```python
from build123d import *

# Parameters (mm, degrees)
F0_W          = 400
F0_H          = 55.75
F2_W          = 20
F2_H          = 19.3462212823
F3_DEPTH      = 30
F4_R          = 15
F5_DEPTH      = 5
F7_DEPTH      = 13
F9_DEPTH      = 50
F11_DEPTH     = 12
F12_R         = 6
F13_DEPTH     = 40
F14_T1_DEPTH  = 63
F14_T3_DEPTH  = 10
F14_S7_W      = 5.1
F14_S7_H      = 5.1
F14_T8_DEPTH  = 5.1
F14_S13_W     = 5.1
F14_S13_H     = 5.1
F14_T14_DEPTH = 5.1
F14_T20_DEPTH = 51
F14_T25_DEPTH = 51


# Not quite as in the source:
# - a fillet or chamfer that OpenCascade refuses, or shapes differently, is made with other operations: its cross-section is extruded or revolved along the edge and cut away or added
# - a pattern or mirror of a feature is missing from the dataset's text; its kind, count and spacing are read off the source's solid


with BuildPart() as f1:
    # F0 (on Front) → F1 (revolve)
    with BuildSketch(Plane.XZ):
        with Locations((0, 27.875)):
            Rectangle(F0_W, F0_H)
        with BuildLine():
            ThreePointArc((200, 55.75), (0, 56.5), (-200, 55.75))
            Line((-200, 55.75), (200, 55.75))
        make_face()
    revolve(axis=Axis((0, 0, 0), (1, 0, 0)))

    # F2 (on face) → F3 (join)
    with BuildSketch(Plane(origin=(-200, 0, 0), x_dir=(0, -1, 0), z_dir=(-1, 0, 0))):
        Rectangle(F2_W, F2_H)
        with BuildLine():
            ThreePointArc((-10, -9.6731106412), (0, -12.5), (10, -9.6731106412))
            Line((10, -9.6731106412), (-10, -9.6731106412))
        make_face()
        with BuildLine():
            Line((-10, 9.6731106412), (10, 9.6731106412))
            ThreePointArc((10, 9.6731106412), (0, 12.5), (-10, 9.6731106412))
        make_face()
    f3 = extrude(amount=F3_DEPTH)

    # F3_copies: F3 across plane
    add(f3.mirror(Plane(origin=(0, 0, 0), x_dir=(0, 0, 1), z_dir=(1, 0, 0))))

    # F4 (on face) → F5 (join)
    with BuildSketch(Plane(origin=(-200, 0, 0), x_dir=(0, -1, 0), z_dir=(-1, 0, 0))):
        Circle(F4_R)
        with BuildLine():
            Line((10, 9.6731106412), (10, -9.6731106412))
            ThreePointArc((10, -9.6731106412), (0, -12.5), (-10, -9.6731106412))
            Line((-10, -9.6731106412), (-10, 9.6731106412))
            ThreePointArc((-10, 9.6731106412), (0, 12.5), (10, 9.6731106412))
        make_face(mode=Mode.SUBTRACT)
    f5 = extrude(amount=F5_DEPTH)

    # F5_copies: F5 across plane
    add(f5.mirror(Plane(origin=(0, 0, 0), x_dir=(0, 0, 1), z_dir=(1, 0, 0))))

    # F6 (on face) → F7 (join)
    with BuildSketch(Plane(origin=(-230, 0, 0), x_dir=(0, -1, 0), z_dir=(-1, 0, 0))):
        Polygon((10, 0.6794919243), (5.1961524227, 9), (-5.1961524227, 9), (-10, 0.6794919243), (-10, -0.6794919243), (-5.1961524227, -9), (5.1961524227, -9), (10, -0.6794919243), align=None)
    extrude(amount=F7_DEPTH)

    # F8 (on face) → F9 (join)
    with BuildSketch(Plane.XY.offset(9)):
        Polygon((-243, 10), (-269, 10), (-269, -10), (-243, -10), (-243, -5.1961524227), (-243, 5.1961524227), align=None)
    extrude(amount=-F9_DEPTH)

    # F10 (on face) → F11 (cut)
    with BuildSketch(Plane(origin=(0, 0, -41), x_dir=(1, 0, 0), z_dir=(0, 0, -1))):
        Polygon((-269, -10), (-259.1794919243, -10), (-267.5, -5.1961524227), (-267.5, 5.1961524227), (-259.1794919243, 10), (-269, 10), align=None)
        Polygon((-257.8205080757, -10), (-243, -10), (-243, 10), (-257.8205080757, 10), (-249.5, 5.1961524227), (-249.5, -5.1961524227), align=None)
    extrude(amount=-F11_DEPTH, mode=Mode.SUBTRACT)

    # F12 (on face) → F13 (join)
    with BuildSketch(Plane(origin=(0, 0, -41), x_dir=(1, 0, 0), z_dir=(0, 0, -1))):
        with Locations((-258.5, 0)):
            Circle(F12_R)
    extrude(amount=F13_DEPTH)

    # F14: fillet of radius 5 on 5 edges, made by hand

    # F14_s2 → F14_t1 (cut)
    with BuildSketch(Plane.XY.offset(-59)):
        with BuildLine():
            ThreePointArc((-269, -5), (-267.5355339059, -8.5355339059), (-264, -10))
            Line((-264, -10), (-264, -10.1))
            Line((-264, -10.1), (-269.1, -10.1))
            Line((-269.1, -10.1), (-269.1, -5))
            Line((-269.1, -5), (-269, -5))
        make_face()
        with BuildLine():
            ThreePointArc((-264, 10), (-267.5355339059, 8.5355339059), (-269, 5))
            Line((-269, 5), (-269.1, 5))
            Line((-269.1, 5), (-269.1, 10.1))
            Line((-269.1, 10.1), (-264, 10.1))
            Line((-264, 10.1), (-264, 10))
        make_face()
    extrude(amount=F14_T1_DEPTH, mode=Mode.SUBTRACT)

    # F14_s4 → F14_t3 (cut)
    with BuildSketch(Plane.XZ.offset(-5)):
        with BuildLine():
            ThreePointArc((-264, 9), (-267.5355339059, 7.5355339059), (-269, 4))
            Line((-269, 4), (-269.1, 4))
            Line((-269.1, 4), (-269.1, 9.1))
            Line((-269.1, 9.1), (-264, 9.1))
            Line((-264, 9.1), (-264, 9))
        make_face()
    extrude(amount=F14_T3_DEPTH, mode=Mode.SUBTRACT)


with BuildPart() as f14_tool6:
    # F14_s7 → F14_t8 (new body)
    with BuildSketch(Plane.XZ.offset(5)):
        with Locations((-266.55, 6.55)):
            Rectangle(F14_S7_W, F14_S7_H)
    extrude(amount=F14_T8_DEPTH)

    # F14_s9 → F14_t10 (revolve, cut)
    with BuildSketch(Plane(origin=(-264, -5, 4), x_dir=(0.7071067812, 0, -0.7071067812), z_dir=(-0.7071067812, 0, -0.7071067812))):
        with BuildLine():
            ThreePointArc((0, -5), (5, 0), (0, 5))
            Line((0, 5), (0, -5))
        make_face()
    revolve(axis=Axis((-264, -5, 4), (0, -1, 0)), mode=Mode.SUBTRACT)


with BuildPart() as f1_1:
    add(f1.part)

    # F14_t5: cut F14_tool6
    add(f14_tool6.part, mode=Mode.SUBTRACT)


with BuildPart() as f14_tool12:
    # F14_s13 → F14_t14 (new body)
    with BuildSketch(Plane.XZ.offset(-5)):
        with Locations((-266.55, 6.55)):
            Rectangle(F14_S13_W, F14_S13_H)
    extrude(amount=-F14_T14_DEPTH)

    # F14_s15 → F14_t16 (revolve, cut)
    with BuildSketch(Plane(origin=(-264, 5, 4), x_dir=(0.7071067812, 0, -0.7071067812), z_dir=(0.7071067812, 0, 0.7071067812))):
        with BuildLine():
            ThreePointArc((0, -5), (5, 0), (0, 5))
            Line((0, 5), (0, -5))
        make_face()
    revolve(axis=Axis((-264, 5, 4), (0, 1, 0)), mode=Mode.SUBTRACT)


with BuildPart() as f1_2:
    add(f1_1.part)

    # F14_t11: cut F14_tool12
    add(f14_tool12.part, mode=Mode.SUBTRACT)


with BuildPart() as f14_tool18:
    # F14_s19 → F14_t20 (new body)
    with BuildSketch(Plane.YZ.offset(-264)):
        with BuildLine():
            ThreePointArc((-5, 9), (-8.5355339059, 7.5355339059), (-10, 4))
            Line((-10, 4), (-10.1, 4))
            Line((-10.1, 4), (-10.1, 9.1))
            Line((-10.1, 9.1), (-5, 9.1))
            Line((-5, 9.1), (-5, 9))
        make_face()
    extrude(amount=F14_T20_DEPTH)

    split(bisect_by=Plane.YZ.offset(-230), keep=Keep.BOTTOM)


with BuildPart() as f1_3:
    add(f1_2.part)

    # F14_t17: cut F14_tool18
    add(f14_tool18.part, mode=Mode.SUBTRACT)


with BuildPart() as f14_tool23:
    # F14_s24 → F14_t25 (new body)
    with BuildSketch(Plane.YZ.offset(-213)):
        with BuildLine():
            ThreePointArc((10, 4), (8.5355339059, 7.5355339059), (5, 9))
            Line((5, 9), (5, 9.1))
            Line((5, 9.1), (10.1, 9.1))
            Line((10.1, 9.1), (10.1, 4))
            Line((10.1, 4), (10, 4))
        make_face()
    extrude(amount=-F14_T25_DEPTH)

    split(bisect_by=Plane.YZ.offset(-230), keep=Keep.BOTTOM)


with BuildPart() as f1_4:
    add(f1_3.part)

    # F14_t22: cut F14_tool23
    add(f14_tool23.part, mode=Mode.SUBTRACT)


solid = f1_4.part
```
Geometry check sheet. Reference: the model listing, model coordinates, mm. A direction names the side the tool comes from. Round coordinates to 2 decimals unless told otherwise and drop trailing zeros. Loops run counter-clockwise (first coordinate to the right, second up) from the corner with the lowest first, then second, coordinate; pieces in that order, holes last. Notation, with made-up numbers: (67, 15) -> (96, 15) arc R20 ccw to (96, 30) -> close; hole circle Ø3 at (31, 47.25). An arc over 180 degrees is marked (long way). Use a Markdown table: item, result.
(1) Mould release check, pull along X, two halves, no side actions. Record for faces 6 (the flat face through (230, 0, 0)), 7 (the flat face through (-247, 0, -29)), 8 (the flat face through (-269, 0, -12)), 9 (the flat face through (-259, 0, -81)): released by +X, released by -X, zero draft, split by the parting line, or undercut.
Calculated:
| item | result |
|---|---|
| face 6 | released by +X |
| face 7 | undercut |
| face 8 | released by -X |
| face 9 | zero draft |
(2) Sectioned sample at A-A (z = -65). Enter the section's corners in (x, y), then the cut area to 3 significant figures.
Calculated:
| item | result |
|---|---|
| outline | circle Ø12 at (-258.5, 0) |
| area | 113 mm² |
(3) Set-up check for faces 1 (the flat face through (-263.398, -7.564, -35.084)), 2 (the cylindrical face through (-252.777, -1.802, -60.72)), 3 (the flat face through (-236.409, -7.633, 4.78)), 4 (the flat face through (217, 10, 0)), 5 (the flat face through (-236.409, -7.564, -4.898)): record each of +Z, -Z, +X, -X, +Y, -Y from which the full face is reachable in a straight line by a thin tool's end or side.
Calculated:
| item | result |
|---|---|
| face 1 | -Z, -X, -Y |
| face 2 | -Z |
| face 3 | +Z, -Y |
| face 4 | +Z, -Z, +X, +Y |
| face 5 | -Z, -Y |
(4) Scan lines: probe 1 along X at (y, z) = (-3.5, -12); probe 2 along X at (y, z) = (42.5, -7); probe 3 along Y at (x, z) = (196, 0). Record each from-to range of solid material in increasing order.
Calculated:
| item | result |
|---|---|
| probe 1 | -269 to -243, -230 to 230 |
| probe 2 | -200 to 200 |
| probe 3 | -55.78 to 55.78 |
(5) Go/stop test with flat-tipped pins: P1, Ø10, axis at y = 1, z = -19.5, coming from the +X side; P2, Ø3, axis at y = -2, z = -37, coming from the +X side; P3, Ø11.5, axis at y = -0.5, z = -37.5, coming from the -X side; P4, Ø10, axis at y = -3, z = 12.5, coming from the +X side. Record where each tip stops, or that it passes through.
Calculated:
| item | result |
|---|---|
| P1 | x = 205 |
| P2 | x = 200 |
| P3 | x = -267.5 |
| P4 | x = 230 |
